Geometry check sheet. Reference: drawing and pictorial views, mm from the part's lowest x, y, z. A direction names the side the tool comes from. Round coordinates to 2 decimals unless told otherwise and drop trailing zeros. Write each loop counter-clockwise with the first axis right and the second up, starting at its lowest first coordinate (ties: lowest second). Pieces come first, ordered by that corner, then holes. Notation, with made-up numbers: M 84.5,52.5 L 136.5,52.5 A16 ccw 136.5,73.5 Z; hole C 19,11 d5. An arc over 180 degrees is marked long. Answer in a Markdown table with one row per item. Add a question column.
1. Sectioned sample at B-B on x = 19.75. Record the cut outline in (y, z), plus the area to 3 significant figures.
2. Material ranges on probe 1 along X at (y, z) = (8.75, 10.5); probe 2 along Z at (x, y) = (17.25, 3.75); probe 3 along X at (y, z) = (12, 3.5), recorded low to high.
3. Set-up check for the marked faces 4 and 5: record each of +Z, -Z, +X, -X, +Y, -Y from which the full face is reachable in a straight line by a thin tool's end or side.
4. Draft check along Z on the marked faces 1, 2 and 3. Enter one of: pulls with the +Z half, pulls with the -Z half, needs draft (parallel to the pull), parting line crosses it, or undercut.
5. Sectioned sample at C-C on z = 10. Record the cut outline in (x, y).
6. Sectioned sample at A-A on y = 4. Record the cut outline in (x, z).
7. Sectioned sample at D-D on y = 11.5. Record the cut outline in (x, z), plus the area to 3 significant figures.
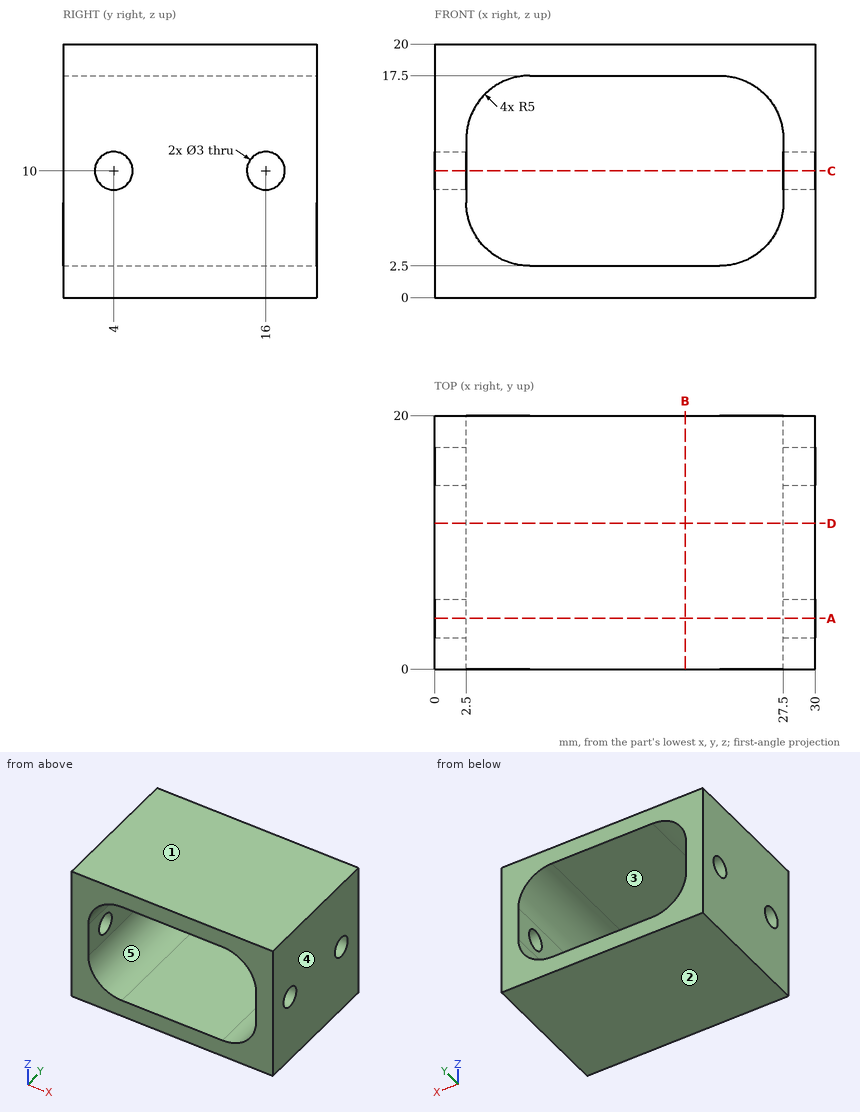
Geometry check:
| question | item | result |
|---|---|---|
| 1 | outline | M 0,0 L 20,0 L 20,2.5 L 0,2.5 Z; M 0,17.5 L 20,17.5 L 20,20 L 0,20 Z |
| 1 | area | 100 mm2 |
| 2 | probe 1 | x = 0 to 2.5, 27.5 to 30 |
| 2 | probe 2 | z = 0 to 2.5, 17.5 to 20 |
| 2 | probe 3 | x = 0 to 4.5, 25.5 to 30 |
| 3 | face 4 | +Z, -Z, +X, +Y, -Y |
| 3 | face 5 | +Y, -Y |
| 4 | face 1 | pulls with the +Z half |
| 4 | face 2 | pulls with the -Z half |
| 4 | face 3 | undercut |
| 5 | outline | M 0,0 L 2.5,0 L 2.5,2.5 L 0,2.5 Z; M 0,5.5 L 2.5,5.5 L 2.5,14.5 L 0,14.5 Z; M 0,17.5 L 2.5,17.5 L 2.5,20 L 0,20 Z; M 27.5,0 L 30,0 L 30,2.5 L 27.5,2.5 Z; M 27.5,5.5 L 30,5.5 L 30,14.5 L 27.5,14.5 Z; M 27.5,17.5 L 30,17.5 L 30,20 L 27.5,20 Z |
| 6 | outline | M 0,0 L 30,0 L 30,8.5 L 27.5,8.5 L 27.5,7.5 A5 cw 22.5,2.5 L 7.5,2.5 A5 cw 2.5,7.5 L 2.5,8.5 L 0,8.5 Z; M 0,11.5 L 2.5,11.5 L 2.5,12.5 A5 cw 7.5,17.5 L 22.5,17.5 A5 cw 27.5,12.5 L 27.5,11.5 L 30,11.5 L 30,20 L 0,20 Z |
| 7 | outline | M 0,0 L 30,0 L 30,20 L 0,20 Z; hole M 2.5,7.5 A5 ccw 7.5,2.5 L 22.5,2.5 A5 ccw 27.5,7.5 L 27.5,12.5 A5 ccw 22.5,17.5 L 7.5,17.5 A5 ccw 2.5,12.5 Z |
| 7 | area | 246 mm2 |
